CAD build for the part. Positions are in the model's coordinates, mm. Face numbers are marked on the shaded views. A direction names the side the tool comes from. Give positions to 0.01 mm unless a question says otherwise; leave off trailing zeros. Loops run counter-clockwise (first coordinate to the right, second up) from the corner with the lowest first, then second, coordinate; pieces in that order, holes last. Notation, with made-up numbers: (81, 22) -> (125, 22) arc R30 cw to (125, 58) -> close; hole circle Ø9 at (51.25, 9.5). An arc over 180 degrees is marked (long way). Write each question's results on one line, items separated by ' | '. Start each with the question number.
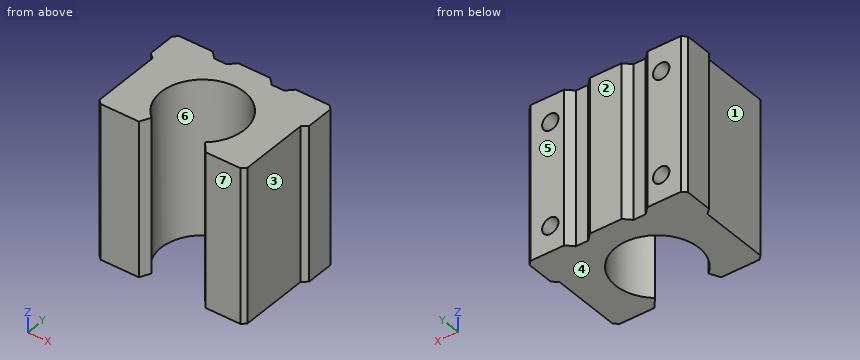
Autodesk Inventor part; units mm, degrees
ref_plane "YZ Plane" through (0, 0, 0) normal (1, 0, 0) x (0, 1, 0)
ref_plane "XZ Plane" through (0, 0, 0) normal (0, 1, 0) x (-1, 0, 0)
ref_plane "XY Plane" through (0, 0, 0) normal (0, 0, 1) x (1, 0, 0)
sketch "Esboço1" plane through (0, 0, 0) normal (0, 0, 1) x (1, 0, 0)
  arc A0 (19.1365, -5.3084) -> (5.6379, -5.3084) centre (12.3872, 2.735) ccw
  line L0 (12.3872, 2.735) -> (12.3872, 19.735) construction
  line L1 (32.3872, 18.735) -> (32.3872, 11.735)
  line L2 (-7.6128, 11.735) -> (-7.6128, 18.735)
  circle A1 centre (12.3872, 2.735) radius 4.25 construction
  line L3 (30.0707, -7.865) -> (21.2817, -7.865)
  line L4 (4.3872, -7.865) -> (-5.2963, -7.865)
  line L5 (5.6379, -5.3084) -> (4.3872, -7.865)
  line L6 (19.1365, -5.3084) -> (21.2817, -7.865)
  line L7 (-7.6128, 11.735) -> (-6.2963, 10.6304)
  line L8 (-6.2963, 10.6304) -> (-6.2963, -6.865)
  line L9 (-1.6128, -7.865) -> (-1.6128, 19.735) construction
  line L10 (26.3872, -7.865) -> (26.3872, 19.735) construction
  line L11 (12.3872, 19.735) -> (12.3872, -10.9717) construction
  line L12 (32.3872, 11.735) -> (31.0707, 10.6304)
  line L13 (31.0707, 10.6304) -> (31.0707, -6.865)
  line L14 (1.3434, 19.735) -> (5.648, 19.735) construction
  line L15 (1.8977, 19.735) -> (3.5675, 18.0653)
  line L16 (0.2217, 19.735) -> (2.5831, 19.735) construction
  line L17 (3.5675, 18.0653) -> (6.6886, 18.0653)
  line L18 (6.6886, 18.0653) -> (8.3584, 19.735)
  line L19 (22.8767, 19.735) -> (21.2069, 18.0653)
  line L20 (21.2069, 18.0653) -> (18.0858, 18.0653)
  line L21 (18.0858, 18.0653) -> (16.416, 19.735)
  line L22 (-6.6128, 19.735) -> (1.8977, 19.735)
  line L23 (8.3584, 19.735) -> (16.416, 19.735)
  line L24 (22.8767, 19.735) -> (31.3872, 19.735)
  line L25 (-7.6128, 18.735) -> (-6.6128, 19.735)
  line L26 (-6.2963, -6.865) -> (-5.2963, -7.865)
  line L27 (30.0707, -7.865) -> (31.0707, -6.865)
  line L28 (32.3872, 18.735) -> (31.3872, 19.735)
  point P0 (0, 0)
  point P1 (-7.6128, 19.735)
  point P2 (32.3872, 19.735)
  point P3 (-6.2963, -7.865)
  point P4 (31.0707, -7.865)
  dimension "d0" = 17
  dimension "d2" = 40
  dimension "d4" = 8.5
  dimension "d6" = 20
  dimension "d10" = 8
  dimension "d12" = 14
  dimension "d13" = 14
  dimension "d19" = 1
  dimension "d20" = 1
  dimension "d21" = 1
  dimension "d22" = 1
  dimension "d23" = 1
  dimension "d24" = 1
  dimension "d25" = 1
  dimension "d26" = 1
extrude "Extrusão1" add sketch "Esboço1" against normal blind 39
sketch "Esboço2" plane through (-6.6128, 19.735, 0) normal (0, 1, 0) x (1, 0, 0)
  line L0 (-1, 0) -> (0.3165, 0)
  line L1 (39, 0) -> (39, 39)
  line L2 (-1, 0) -> (39, 0)
  line L3 (39, 0) -> (39, 39)
  line L4 (39, 39) -> (-1, 39)
  line L5 (-1, 0) -> (-1, 39)
  line L6 (-1, 39) -> (-1, 0)
  line L7 (8.5105, 0) -> (0, 0)
  line L8 (11, 39) -> (1.3165, 39)
  line L9 (27.8945, 0) -> (36.6835, 0)
  line L10 (33, 0) -> (33, 39) construction
  line L11 (29.5, 0) -> (8.5, 0)
  line L12 (19, 0) -> (19, 39) construction
  line L13 (8.5, 39) -> (29.5, 39)
  line L14 (11, 39) -> (1.3165, 39)
  line L15 (5, 39) -> (5, 0) construction
  line L16 (1.3165, 0) -> (11, 0)
  line L17 (-4.598, 19.5) -> (42.402, 19.5) construction
  line L18 (-10.187, 32.5) -> (53.6518, 32.5) construction
  line L19 (-10.187, 6.5) -> (53.6518, 6.5) construction
  circle A0 centre (5, 32.5) radius 1.6801 construction
  circle A1 centre (33, 32.5) radius 1.5751 construction
  circle A2 centre (5, 6.5) radius 1.6801 construction
  circle A3 centre (33, 6.5) radius 1.5751 construction
  point P0 (6.6128, 0)
  point P1 (12.2507, 0)
  point P2 (25.7493, 0)
  point P3 (25.7493, 39)
  point P4 (12.2507, 39)
  dimension "d29" = 14
  dimension "d31" = 14
  dimension "d32" = 47
  dimension "d33" = 13
  dimension "d34" = 13
hole "Furo1" at (-1.6128, 19.735, -32.5) at (26.3872, 19.735, -32.5) at (26.3872, 19.735, -6.5) at (-1.6128, 19.735, -6.5) direction (0, -1, 0) diameter 4.134 depth 14.2 tip angle 118
properties part number "PilowBlockAberto"
Q1. Mould opens along Y. For the marked faces 4, 5, 6 and 7 say: pulls with the +Y half, pulls with the -Y half, needs draft (parallel to the pull), parting line crosses it, or undercut.
Q2. Saw through at C-C, the plane y = -1.75. List the corners of the cut face in (x, z).
Q3. Wall check: L1, parallel to X at y = 14.25, z = -32.5; L2, parallel to X at y = 10, z = -32.5; L3, parallel to X at y = 3, z = -12.5. Give the ranges that are in metal, low to high.
Q4. Which spindle directions (+Z, -Z, +X, -X, +Y, -Y) get a long thin tool onto all of the face, cutting with end or side? Do the marked faces 1, 2 and 3. Say none if no direction does.
Q5. Saw through at A-A, the plane y = 9.25. List the corners of the cut face in (x, z), then the cut area to 3 significant figures.
Q6. Saw through at B-B, the plane z = -9.5. List the corners of the cut face in (x, y) (1 decimal), then the cut area to 3 significant figures.
Q7. Saw through at D-D, the plane x = 10.5. List the corners of the cut face in (y, z) (3 decimals), then the cut area to 3 significant figures.
Q8. Drop flat-ended pins along their axis: pin 1 (5 mm diameter, centred on y = -2.5, z = -22, fed in from +X); pin 2 (2 mm diameter, centred on x = 5.5, z = -32.5, fed in from +Y); pin 3 (2.5 mm diameter, centred on x = 6, z = -13, fed in from +Y). Give the stop position or say it passes through.
Answer block:
1) face 4: needs draft | face 5: pulls with the +Y half | face 6: undercut | face 7: pulls with the -Y half
2) outline: (-6.3, -39) -> (2.89, -39) -> (2.89, 0) -> (-6.3, 0) -> close; (21.88, -39) -> (31.07, -39) -> (31.07, 0) -> (21.88, 0) -> close
3) L1: x = -7.61 to -3.68, 0.45 to 24.32, 28.45 to 32.39 | L2: x = -6.3 to -3.68, 0.45 to 4.81, 19.97 to 24.32, 28.45 to 31.07 | L3: x = -6.3 to 1.89, 22.88 to 31.07
4) face 1: +Z, -Z, -X, -Y | face 2: +Z, -Z, +X, -X, +Y | face 3: +Z, -Z, +X, -Y
5) outline: (-6.3, -39) -> (4.15, -39) -> (4.15, 0) -> (-6.3, 0) -> close; (20.62, -39) -> (31.07, -39) -> (31.07, 0) -> (20.62, 0) -> close; hole circle Ø4.13 at (-1.61, -32.5); hole circle Ø4.13 at (-1.61, -6.5); hole circle Ø4.13 at (26.39, -32.5); hole circle Ø4.13 at (26.39, -6.5) | area: 761 mm2
6) outline: (-7.6, 11.7) -> (-6.3, 10.6) -> (-6.3, -6.9) -> (-5.3, -7.9) -> (4.4, -7.9) -> (5.6, -5.3) arc R10.5 cw (long way) to (19.1, -5.3) -> (21.3, -7.9) -> (30.1, -7.9) -> (31.1, -6.9) -> (31.1, 10.6) -> (32.4, 11.7) -> (32.4, 18.7) -> (31.4, 19.7) -> (22.9, 19.7) -> (21.2, 18.1) -> (18.1, 18.1) -> (16.4, 19.7) -> (8.4, 19.7) -> (6.7, 18.1) -> (3.6, 18.1) -> (1.9, 19.7) -> (-6.6, 19.7) -> (-7.6, 18.7) -> close | area: 673 mm2
7) outline: (13.064, -39) -> (19.735, -39) -> (19.735, 0) -> (13.064, 0) -> close | area: 260 mm2
8) pin 1: stops at x = 31.07 | pin 2: stops at y = 18.07 | pin 3: stops at y = 18.63
